Here's how the part is built. I have some questions about the finished solid (model axes, mm). Give positions to 0.01 mm unless a question says otherwise; leave off trailing zeros. Write each loop counter-clockwise with the first axis right and the second up, starting at its lowest first coordinate (ties: lowest second). Pieces come first, ordered by that corner, then holes. Notation, with made-up numbers: (17.25, 10) -> (21.25, 10) arc R31 ccw to (21.25, 35) -> close; hole circle Ø3 at (-12, 22.5). An arc over 180 degrees is marked (long way). Answer as CSV lines item,"result". Start each with the question number.
Solid Edge part; units mm, degrees
sketch "Sketch1" plane through (0, 0, 0) normal (0, 0, 1) x (1, 0, 0)
  line L0 (0, 0) -> (-170.02, 0)
  line L1 (-170.02, 0) -> (-170.02, -85)
  line L2 (-170.02, -85) -> (0, -85)
  line L3 (0, -85) -> (0, 0)
extrude "Protrusion1" add sketch "Sketch1" against normal blind 20.4
chamfer "Chamfer_2" [suppressed]
chamfer "Chamfer_3" [suppressed]
chamfer "Chamfer_9" [suppressed]
chamfer "Chamfer_10" [suppressed]
sketch "Sketch2" plane through (-85.01, -42.5, 0) normal (0, 0, 1) x (1, 0, 0)
  circle A0 centre (-42.49, -7) radius 6.65
  circle A1 centre (42.51, -7) radius 6.65
extrude "ExtrudedCutout_4" cut sketch "Sketch2" against normal blind 22
sketch "Sketch3" plane through (-85.01, -42.5, 0) normal (0, 0, 1) x (1, 0, 0)
  circle A0 centre (-120.01, -7) radius 57.5
  circle A1 centre (120.01, -7) radius 57.5
extrude "ExtrudedCutout_5" cut sketch "Sketch3" against normal blind 22
chamfer "Chamfer_14" distance 3 distance2 1 1 edges at (0, 0, -10.2) measured on face at (0, -3.2715, -16.796)
chamfer "Chamfer_15" distance 3 distance2 1 1 edges at (-170.02, 0, -10.2) measured on face at (-170.02, -0.6078, -16.796)
chamfer "Chamfer_16" distance 2.2 angle 63 1 edges at (-159.7873, -85, -10.2) measured on face at (-136.3571, -85, -16.796)
chamfer "Chamfer_17" distance 2.2 angle 63 1 edges at (-10.2327, -85, -10.2) measured on face at (-134.5017, -85, -16.796)
Item 1: If we section it at C-C (z = -4): Please give me the cut outline in (x, y).
Item 2: I'm going to push flat-ended pins straight in: pin 1 (1 mm diameter, centred on y = -48.5, z = -10, fed in from +X); pin 2 (6 mm diameter, centred on y = -65, z = -13.5, fed in from +X); pin 3 (4 mm diameter, centred on y = -58.5, z = -15, fed in from -X). Where does each tip first touch, or does it pass through?
Item 3: If we section it at A-A (x = -42.5): Please give me the cut outline in (y, z), and give its area (3 significant figures).
Item 4: If I drill on line 1 (Y direction, x = -127.5, z = -13.75); line 2 (Y direction, x = -152, z = -19.5); line 3 (X direction, y = -33, z = -17.5), over which ranges is the centre line in solid material (lowest first)? Write a range as [from, to].
Item 5: If we section it at D-D (x = -125.5): Please give me the cut outline in (y, z).
Item 6: We'd pull the mould along Y, two halves only. Please class faces 1 (the face through (-36.36, -52.05, -10.06)), 2 (the face through (-86, -85, -10)), 3 (the face through (-86, -42, 0)): released by +Y, released by -Y, zero draft, split by the parting line, or undercut.
Item 7: If we section it at B-B (y = -49.5): Please give me the cut outline in (x, z).
Final values:
1,outline,"(-170.02, -3.88) arc R57.5 cw to (-158.47, -83.26) -> (-157.59, -85) -> (-12.43, -85) -> (-11.55, -83.26) arc R57.5 cw to (0, -3.88) -> (0, -3) -> (-1, 0) -> (-169.02, 0) -> (-170.02, -3) -> close; hole circle Ø13.3 at (-127.5, -49.5); hole circle Ø13.3 at (-42.5, -49.5)"
2,pin 1,"x = -22.48"
2,pin 2,"x = -19.44"
2,pin 3,"x = -148.58"
3,outline,"(-85, -20.4) -> (-56.15, -20.4) -> (-56.15, 0) -> (-85, 0) -> close; (-42.85, -20.4) -> (0, -20.4) -> (0, 0) -> (-42.85, 0) -> close"
3,area,"1,460 mm2"
4,line 1,"[-85, -56.15], [-42.85, 0]"
4,line 2,"[-85, -71.75], [-27.25, 0]"
4,line 3,"[-149.94, -20.08]"
5,outline,"(-85, -20.4) -> (-55.84, -20.4) -> (-55.84, 0) -> (-85, 0) -> close; (-43.16, -20.4) -> (0, -20.4) -> (0, 0) -> (-43.16, 0) -> close"
6,face 1,"undercut"
6,face 2,"released by -Y"
6,face 3,"zero draft"
7,outline,"(-147.52, -20.4) -> (-134.15, -20.4) -> (-134.15, 0) -> (-147.52, 0) -> close; (-120.85, -20.4) -> (-49.15, -20.4) -> (-49.15, 0) -> (-120.85, 0) -> close; (-35.85, -20.4) -> (-22.5, -20.4) -> (-22.5, 0) -> (-35.85, 0) -> close"
